Autodesk Inventor part; units mm, degrees
ref_plane "YZ Plane" through (0, 0, 0) normal (1, 0, 0) x (0, 1, 0)
ref_plane "XZ Plane" through (0, 0, 0) normal (0, 1, 0) x (-1, 0, 0)
ref_plane "XY Plane" through (0, 0, 0) normal (0, 0, 1) x (1, 0, 0)
sketch "Sketch1" plane through (0, 0, 0) normal (0, 0, 1) x (1, 0, 0)
  line L0 (0, 0) -> (93, 0)
  line L1 (93, 0) -> (93, 66)
  line L2 (93, 66) -> (0, 66)
  line L3 (0, 66) -> (0, 0)
  dimension "d0" = 93
  dimension "d1" = 66
extrude "Extrusion1" add sketch "Sketch1" along normal blind 2
sketch "Sketch2" plane through (0, 0, 2) normal (0, 0, 1) x (1, 0, 0)
  line L0 (93, 0) -> (93, 66)
  line L1 (93, 66) -> (0, 66)
  line L2 (0, 66) -> (0, 0)
  line L3 (0, 0) -> (93, 0)
  line L4 (0, 70) -> (101, 70)
  line L5 (101, 70) -> (101, -4)
  line L6 (101, -4) -> (0, -4)
  line L7 (0, 66) -> (0, 70)
  line L8 (0, -4) -> (0, 0)
  dimension "d4" = 4
  dimension "d5" = 8
  dimension "d6" = 4
extrude "Extrusion2" add sketch "Sketch2" along normal blind 2
sketch "Sketch3" plane through (0, 0, 0) normal (0, 0, -1) x (-1, 0, 0)
  circle A0 centre (-26.8923, 57.0496) radius 1.375
  circle A1 centre (-84.8923, 57.0496) radius 1.375
  circle A2 centre (-84.8923, 8.0496) radius 1.375
  circle A3 centre (-26.8923, 8.0496) radius 1.375
  point P0 (0, 0)
hole "Hole1" at (26.8923, 57.0496, 0) at (84.8923, 57.0496, 0) at (84.8923, 8.0496, 0) at (26.8923, 8.0496, 0) direction (0, 0, 1) diameter 2.75 depth 4
sketch "Sketch4" plane through (0, 0, 4) normal (0, 0, 1) x (1, 0, 0)
  line L0 (101, 70) -> (0, 70)
  line L1 (0, -4) -> (101, -4)
  line L2 (0, 70) -> (0, -4)
  line L3 (101, -4) -> (101, 70)
  point P0 (0, 0)
  point P1 (97, 33)
  dimension "d16" = 37
  dimension "d18" = 4
hole "Hole2" at (97, 33, 4) direction (0, 0, -1) diameter 4 depth 3
thread "Thread1"
thread "Thread2"
thread "Thread3"
thread "Thread4"
thread "Thread5"
properties part number "Tapa raspberry" material "ABS Plastic"
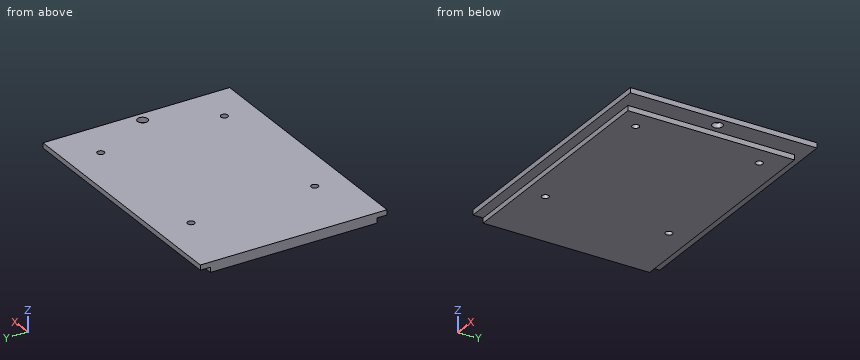
The listing builds one solid part. Answer for the finished solid, in the listing's coordinates (mm). Coordinates: 2 decimals unless noted, no trailing zeros. Write each loop counter-clockwise with the first axis right and the second up, starting at its lowest first coordinate (ties: lowest second). Pieces come first, ordered by that corner, then holes. Notation, with made-up numbers: (5, -6) - (45, -6) arc R18 cw to (45, 19) - close; hole circle Ø2 at (-3, 70). An arc over 180 degrees is marked (long way). One line per item, written item: value.
1) Find section C-C (z = 1.2). Give the vertices of the cut face in (x, y) (3 decimals).
Geometry check:
outline: (0, 0) - (93, 0) - (93, 66) - (0, 66) - close; hole circle Ø2.75 at (26.892, 8.05); hole circle Ø2.75 at (26.892, 57.05); hole circle Ø2.75 at (84.892, 8.05); hole circle Ø2.75 at (84.892, 57.05)
2) Each of these flat-tipped pins is pushed along its axis until it touches: pin 1 Ø3.5 at (x, y) = (97, 33) entering from +Z; pin 2 Ø0.6 at (x, z) = (33.5, 1) entering from -Y; pin 3 Ø0.6 at (x, z) = (68.5, 1) entering from +Y; pin 4 Ø1 at (y, z) = (30, 0.5) entering from +X. Where does it stop, or does it pass through?
Geometry check:
pin 1: passes through
pin 2: stops at y = 0
pin 3: stops at y = 66
pin 4: stops at x = 93
3) Find section D-D (x = 58.5). Give the vertices of the cut face in (y, z).
Geometry check:
outline: (-4, 2) - (0, 2) - (0, 0) - (66, 0) - (66, 2) - (70, 2) - (70, 4) - (-4, 4) - close
4) Consider line 1 along X through (y, z) = (9, 1.05); line 2 along X through (y, z) = (33, 3.65); line 3 along X through (y, z) = (7.5, 2.05). Determine where each line is inside the solid, lowest interval first. Write a range as from..to.
Geometry check:
line 1: x = 0..25.9, 27.89..83.9, 85.89..93
line 2: x = 0..95, 99..101
line 3: x = 0..25.63, 28.15..83.63, 86.15..101
5) Find section B-B (x = 97). Give the vertices of the cut face in (y, z).
Geometry check:
outline: (-4, 2) - (31, 2) - (31, 4) - (-4, 4) - close; (35, 2) - (70, 2) - (70, 4) - (35, 4) - close
6) Find section A-A (y = 33). Give the vertices of the cut face in (x, z), and give its area (3 significant figures).
Geometry check:
outline: (0, 0) - (93, 0) - (93, 2) - (95, 2) - (95, 4) - (0, 4) - close; (99, 2) - (101, 2) - (101, 4) - (99, 4) - close
area: 380 mm2
